from build123d import *

# Parameters (mm, degrees)
SKETCH2_W            = 195
SKETCH2_H            = 180
BOSS_EXTRUDE1_DEPTH  = 50
CUT_EXTRUDE1_DEPTH   = 15
BOSS_EXTRUDE4_DEPTH  = 50
SKETCH14_W           = 70
SKETCH14_H           = 65
SKETCH14_W_2         = 95
BOSS_EXTRUDE8_DEPTH  = 35
SHELL2_OUTLINE_W     = 175
SHELL2_OUTLINE_H     = 65
SHELL2_DEPTH         = 75
SHELL2_2_OUTLINE_W   = 175
SHELL2_2_OUTLINE_H   = 95
SHELL2_2_DEPTH       = 25
SHELL2_START         = 25
SHELL2_3_DEPTH       = 15
SKETCH15_W           = 46
SKETCH15_H           = 21
CUT_EXTRUDE2_DEPTH   = 30
SKETCH16_W           = 46
SKETCH16_H           = 21
CUT_EXTRUDE3_DEPTH   = 30
SKETCH17_W           = 7.5
SKETCH17_H           = 8
BOSS_EXTRUDE9_DEPTH  = 2
SKETCH18_W           = 15
SKETCH18_H           = 2
BOSS_EXTRUDE10_DEPTH = 15
SKETCH19_W           = 33
SKETCH19_H           = 29
CUT_EXTRUDE14_DEPTH  = 10


# Read off the part's stored shape, not the designer's step: Shell2
with BuildPart() as part:
    # Sketch2 → Boss-Extrude1 (new body)
    with BuildSketch(Plane(origin=(0, 0, 0), x_dir=(1, 0, 0), z_dir=(0, 1, 0))):
        with Locations((97.5, 90)):
            Rectangle(SKETCH2_W, SKETCH2_H)
    extrude(amount=BOSS_EXTRUDE1_DEPTH)

    # Sketch3 → Cut-Extrude1 (cut)
    with BuildSketch(Plane(origin=(0, 50, 0), x_dir=(1, 0, 0), z_dir=(0, 1, 0))):
        with BuildLine():
            Line((90, 12), (90, 73))
            ThreePointArc((90, 73), (90.585786438, 74.414213562), (92, 75))
            Line((92, 75), (183, 75))
            ThreePointArc((183, 75), (184.414213562, 74.414213562), (185, 73))
            Line((185, 73), (185, 12))
            ThreePointArc((185, 12), (184.414213562, 10.585786438), (183, 10))
            Line((183, 10), (92, 10))
            ThreePointArc((92, 10), (90.585786438, 10.585786438), (90, 12))
        make_face()
        with BuildLine():
            Line((12, 10), (78, 10))
            ThreePointArc((78, 10), (79.414213562, 10.585786438), (80, 12))
            Line((80, 12), (80, 73))
            ThreePointArc((80, 73), (79.414213562, 74.414213562), (78, 75))
            Line((78, 75), (12, 75))
            ThreePointArc((12, 75), (10.585786438, 74.414213562), (10, 73))
            Line((10, 73), (10, 12))
            ThreePointArc((10, 12), (10.585786438, 10.585786438), (12, 10))
        make_face()
    extrude(amount=-CUT_EXTRUDE1_DEPTH, mode=Mode.SUBTRACT)

    # Sketch6 → Boss-Extrude4 (add)
    with BuildSketch(Plane(origin=(0, 50, 0), x_dir=(1, 0, 0), z_dir=(0, 1, 0))):
        Polygon((0, 180), (185, 180), (195, 180), (195, 95), (185, 95), (0, 95), align=None)
        with BuildLine():
            Line((185, 168), (185, 107))
            ThreePointArc((185, 107), (184.414213562, 105.585786438), (183, 105))
            Line((183, 105), (92, 105))
            ThreePointArc((92, 105), (90.585786438, 105.585786438), (90, 107))
            Line((90, 107), (90, 168))
            ThreePointArc((90, 168), (90.585786438, 169.414213562), (92, 170))
            Line((92, 170), (183, 170))
            ThreePointArc((183, 170), (184.414213562, 169.414213562), (185, 168))
        make_face(mode=Mode.SUBTRACT)
        with BuildLine():
            Line((80, 107), (80, 168))
            ThreePointArc((80, 168), (79.414213562, 169.414213562), (78, 170))
            Line((78, 170), (12, 170))
            ThreePointArc((12, 170), (10.585786438, 169.414213562), (10, 168))
            Line((10, 168), (10, 107))
            ThreePointArc((10, 107), (10.585786438, 105.585786438), (12, 105))
            Line((12, 105), (78, 105))
            ThreePointArc((78, 105), (79.414213562, 105.585786438), (80, 107))
        make_face(mode=Mode.SUBTRACT)
    extrude(amount=BOSS_EXTRUDE4_DEPTH)

    # Sketch14 → Boss-Extrude8 (add)
    with BuildSketch(Plane(origin=(0, 50, 0), x_dir=(1, 0, 0), z_dir=(0, 1, 0))):
        with Locations((45, 137.5)):
            Rectangle(SKETCH14_W, SKETCH14_H)
        with Locations((137.5, 137.5)):
            Rectangle(SKETCH14_W_2, SKETCH14_H)
    extrude(amount=BOSS_EXTRUDE8_DEPTH)

    # Shell2 outline → Shell2 (cut)
    with BuildSketch(Plane(origin=(0, 0, 0), x_dir=(1, 0, 0), z_dir=(0, 1, 0))):
        with Locations((97.5, 137.5)):
            Rectangle(SHELL2_OUTLINE_W, SHELL2_OUTLINE_H)
    extrude(amount=SHELL2_DEPTH, mode=Mode.SUBTRACT)

    # Shell2 2 outline → Shell2 2 (cut)
    with BuildSketch(Plane(origin=(0, 0, 0), x_dir=(1, 0, 0), z_dir=(0, 1, 0))):
        with Locations((97.5, 57.5)):
            Rectangle(SHELL2_2_OUTLINE_W, SHELL2_2_OUTLINE_H)
    extrude(amount=SHELL2_2_DEPTH, mode=Mode.SUBTRACT)

    # Shell2 3 outline → Shell2 3 (cut)
    with BuildSketch(Plane(origin=(0, 0, 0), x_dir=(1, 0, 0), z_dir=(0, 1, 0)).offset(SHELL2_START)):
        with BuildLine():
            Line((10, 105), (10, 84.832159566))
            ThreePointArc((10, 84.832159566), (10.996484877, 84.957966273), (12, 85))
            Line((12, 85), (78, 85))
            ThreePointArc((78, 85), (81.676851089, 84.422817781), (85, 82.746794345))
            ThreePointArc((85, 82.746794345), (88.323148911, 84.422817781), (92, 85))
            Line((92, 85), (183, 85))
            ThreePointArc((183, 85), (184.003515123, 84.957966273), (185, 84.832159566))
            Line((185, 84.832159566), (185, 105))
            Line((185, 105), (10, 105))
        make_face()
    extrude(amount=SHELL2_3_DEPTH, mode=Mode.SUBTRACT)

    # SurfaceCut1
    split(bisect_by=Plane(origin=(0, 50, 0), x_dir=(1, 0, 0), z_dir=(0, 1, 0)), keep=Keep.TOP)

    # Sketch15 → Cut-Extrude2 (cut)
    with BuildSketch(Plane(origin=(0, 85, 0), x_dir=(1, 0, 0), z_dir=(0, 1, 0))):
        with Locations((45, 137.5)):
            Rectangle(SKETCH15_W, SKETCH15_H)
    extrude(amount=-CUT_EXTRUDE2_DEPTH, mode=Mode.SUBTRACT)

    # Sketch16 → Cut-Extrude3 (cut)
    with BuildSketch(Plane(origin=(0, 85, 0), x_dir=(1, 0, 0), z_dir=(0, 1, 0))):
        with Locations((137.5, 137.5)):
            Rectangle(SKETCH16_W, SKETCH16_H)
    extrude(amount=-CUT_EXTRUDE3_DEPTH, mode=Mode.SUBTRACT)

    # Sketch17 → Boss-Extrude9 (add)
    with BuildSketch(Plane.XY.offset(-148)):
        with Locations((41.25, 71)):
            Rectangle(SKETCH17_W, SKETCH17_H)
        with Locations((48.75, 71)):
            Rectangle(SKETCH17_W, SKETCH17_H)
    boss_extrude9 = extrude(amount=-BOSS_EXTRUDE9_DEPTH)

    # Sketch18 → Boss-Extrude10 (add)
    with BuildSketch(Plane.XY.offset(-148)):
        with Locations((45, 68)):
            Rectangle(SKETCH18_W, SKETCH18_H)
    boss_extrude10 = extrude(amount=BOSS_EXTRUDE10_DEPTH)

    # Mirror1: Boss-Extrude9, Boss-Extrude10 across plane
    add(boss_extrude9.mirror(Plane.ZY.offset(-91.25)))
    add(boss_extrude10.mirror(Plane.ZY.offset(-91.25)))

    # Sketch19 → Cut-Extrude14 (cut)
    with BuildSketch(Plane.XY.offset(-95)):
        with Locations((45, 69.5)):
            Rectangle(SKETCH19_W, SKETCH19_H)
        with Locations((137.5, 69.5)):
            Rectangle(SKETCH19_W, SKETCH19_H)
    extrude(amount=-CUT_EXTRUDE14_DEPTH, mode=Mode.SUBTRACT)


solid = part.part
Read the model definition and answer for the solid it produces. Units are mm, in the model's axes. A direction names the side the tool comes from. Round coordinates to 2 decimals unless told otherwise and drop trailing zeros. Order: outer loops, then holes, each group sorted by start corner. A loop starts at its lowest first (then second) coordinate and runs counter-clockwise, first axis right, second up.
1) Flat-ended cylindrical pins translate along their axes: pin 1 (5 mm diameter, centred on x = 137.5, z = -141, fed in from +Y); pin 2 (2.5 mm diameter, centred on x = 52.5, y = 78.5, fed in from +Z); pin 3 (12 mm diameter, centred on x = 134, z = -143.5, fed in from -Y). Find the tip coordinate at first contact, or state that the pin passes through.
2) The mould has two halves that part along X. Classify faces 1 (the face through (96, 75, -95)), 2 (the face through (137, 55, -100)): released by +X, released by -X, zero draft, split by the parting line, or undercut.
3) The part is cut by section C-C on y = 60. Write down the section's boundary in (x, z).
4) The part is cut by section D-D on x = 66. Write down the section's boundary in (y, z), plus the area to 3 significant figures.
5) The part is cut by section A-A on y = 72. Write down the section's boundary in (x, z), plus the area to 3 significant figures.
6) For faces 3 (the face through (137, 84, -100)), 4 (the face through (114.5, 80, -137)), 5 (the face through (138, 92, -105)), 6 (the face through (45, 67, -142)), determine the directions among +Z, -Z, +X, -X, +Y, -Y from which every point of the face is accessible in a straight line to the end or side of a thin tool.
7) The part is cut by section B-B on x = 149.5. Write down the section's boundary in (y, z).
8) Straight lines are drawn through the part: L1, parallel to X at y = 95, z = -110; L2, parallel to X at y = 75.5, z = -137; L3, parallel to X at y = 55, z = -115.5. For each, find the intervals that lie inside material, in ascending order.
Resolved:
1. pin 1: stops at y = 69
1. pin 2: stops at z = -105
1. pin 3: stops at y = 67
2. face 1: zero draft
2. face 2: undercut
3. outline: (0, -180) - (195, -180) - (195, -95) - (154, -95) - (154, -105) - (185, -105) - (185, -170) - (10, -170) - (10, -105) - (28.5, -105) - (28.5, -95) - (0, -95) - close; (61.5, -105) - (121, -105) - (121, -95) - (61.5, -95) - close
4. outline: (50, -180) - (100, -180) - (100, -170) - (85, -170) - (85, -148) - (75, -148) - (75, -170) - (50, -170) - close; (50, -105) - (75, -105) - (75, -127) - (85, -127) - (85, -105) - (100, -105) - (100, -95) - (50, -95) - close
4. area: 1,440 mm2
5. outline: (0, -180) - (195, -180) - (195, -95) - (154, -95) - (154, -105) - (185, -105) - (185, -170) - (10, -170) - (10, -105) - (28.5, -105) - (28.5, -95) - (0, -95) - close; (37.5, -150) - (52.5, -150) - (52.5, -148) - (37.5, -148) - close; (61.5, -105) - (121, -105) - (121, -95) - (61.5, -95) - close; (130, -150) - (145, -150) - (145, -148) - (130, -148) - close
5. area: 4,600 mm2
6. face 3: +Z
6. face 4: +Y, -Y
6. face 5: +Y
6. face 6: +Z, -Y
7. outline: (50, -180) - (100, -180) - (100, -170) - (85, -170) - (85, -148) - (75, -148) - (75, -170) - (50, -170) - close; (50, -105) - (55, -105) - (55, -95) - (50, -95) - close; (75, -127) - (85, -127) - (85, -105) - (100, -105) - (100, -95) - (84, -95) - (84, -105) - (75, -105) - close
8. L1: x = 0 to 10, 80 to 90, 185 to 195
8. L2: x = 0 to 22, 68 to 114.5, 160.5 to 195
8. L3: x = 0 to 10, 185 to 195
